```python
from build123d import *

# Parameters (mm, degrees)
BOSS_EXTRUDE1_DEPTH = 27.94
SKETCH2_R           = 3.175
BOSS_EXTRUDE2_DEPTH = 2.54
BOSS_EXTRUDE3_START = 3.81
SKETCH3_W           = 27.611756562
SKETCH3_H           = 25.107614127
SKETCH3_R           = 3.175
BOSS_EXTRUDE3_DEPTH = 3.81
SKETCH4_R           = 3.175
BOSS_EXTRUDE4_DEPTH = 18.954575182
SKETCH5_W           = 22.86
SKETCH5_H           = 21.59
CUT_EXTRUDE1_DEPTH  = 564.927995542


with BuildPart() as part:
    # Sketch1 → Boss-Extrude1 (new body)
    with BuildSketch(Plane.XY):
        with BuildLine():
            Line((-518.959059009, 348.633589309), (-527.727560082, 348.633589309))
            Line((-527.727560082, 348.633589309), (-527.727560082, 323.525975182))
            Line((-527.727560082, 323.525975182), (-500.11580352, 323.525975182))
            Line((-500.11580352, 323.525975182), (-500.11580352, 330.828951218))
            Line((-500.11580352, 330.828951218), (-503.31589155, 328.989459324))
            ThreePointArc((-503.31589155, 328.989459324), (-505.910190066, 327.86159111), (-508.689794246, 327.335975182))
            ThreePointArc((-508.689794246, 327.335975182), (-520.655570716, 333.67086151), (-520.107560082, 347.198990562))
            ThreePointArc((-520.107560082, 347.198990562), (-519.559291988, 347.937090778), (-518.959059009, 348.633589309))
        make_face()
    extrude(amount=-BOSS_EXTRUDE1_DEPTH)

    # Sketch2 → Boss-Extrude2 (add)
    with BuildSketch(Plane(origin=(0, 0, -25.4), x_dir=(-1, 0, 0), z_dir=(0, 0, -1))):
        with BuildLine():
            Line((500.11580352, 330.828951218), (500.11580352, 348.633589309))
            Line((500.11580352, 348.633589309), (518.959059009, 348.633589309))
            ThreePointArc((518.959059009, 348.633589309), (519.579835197, 332.088638139), (503.31589155, 328.989459324))
            Line((503.31589155, 328.989459324), (500.11580352, 330.828951218))
        make_face()
        with Locations(Location((509.64503004, 340, 0), (0, 0, 180))):
            Circle(SKETCH2_R, mode=Mode.SUBTRACT)
    extrude(amount=BOSS_EXTRUDE2_DEPTH)

    # Sketch3 → Boss-Extrude3 (add)
    with BuildSketch(Plane.XY.offset(BOSS_EXTRUDE3_START)):
        with Locations((-513.921681801, 336.079782246)):
            Rectangle(SKETCH3_W, SKETCH3_H)
        with Locations((-509.64503004, 340)):
            Circle(SKETCH3_R, mode=Mode.SUBTRACT)
    extrude(amount=-BOSS_EXTRUDE3_DEPTH)

    # Sketch4 → Boss-Extrude4 (add)
    with BuildSketch(Plane(origin=(0, 323.525975182, 0), x_dir=(1, 0, 0), z_dir=(0, 1, 0))):
        Polygon((-562.359793246, 33.660212868), (-511.559810801, 33.702445144), (-511.559793246, -29.839787132), (-562.359793246, -29.839787132), align=None)
        with Locations(Location((-539.26913234, -22.159639935, 0), (0, 0, 270))):
            Circle(SKETCH4_R, mode=Mode.SUBTRACT)
        with Locations(Location((-554.645069674, 26.257511479, 0), (0, 0, 270))):
            Circle(SKETCH4_R, mode=Mode.SUBTRACT)
    extrude(amount=-BOSS_EXTRUDE4_DEPTH)

    # Sketch5 → Cut-Extrude1 (cut, through all)
    with BuildSketch(Plane(origin=(0, 323.525975182, 0), x_dir=(1, 0, 0), z_dir=(0, 1, 0))):
        with Locations((-550.929793246, 0.005212868)):
            Rectangle(SKETCH5_W, SKETCH5_H)
    extrude(amount=-CUT_EXTRUDE1_DEPTH, mode=Mode.SUBTRACT)


solid = part.part
```
Geometry: final body of the model. Coordinates: model frame, mm. A direction names the side the tool comes from. Round coordinates to 2 decimals unless told otherwise and drop trailing zeros. Order: outer loops, then holes, each group sorted by start corner. A loop starts at its lowest first (then second) coordinate and runs counter-clockwise, first axis right, second up. Notation, with made-up numbers: M 32.25,77.25 L 83.25,77.25 A20 ccw 83.25,108.25 Z; hole C -37,70 d10. An arc over 180 degrees is marked long. One line per item, written item: value.
(1) Cut plane B-B (z = -2.5). Return the cut outline in (x, y).
Result sheet:
outline: M -539.5,304.57 L -511.56,304.57 L -511.56,323.53 L -500.12,323.53 L -500.12,330.83 L -503.32,328.99 A12.7 cw -518.96,348.63 L -527.73,348.63 L -527.73,323.53 L -539.5,323.53 Z
(2) Reachability of faces 1 (the flat face through (-539.5, 314, 0)), 2 (the flat face through (-514, 336, 3.81)), 3 (the flat face through (-527.728, 336, -12)), 4 (the flat face through (-501.693, 329.922, -12.522)) from +Z, -Z, +X, -X, +Y, -Y: full face, straight path, thin tool, end or side. Return the list, or none.
Result sheet:
face 1: -X, +Y, -Y
face 2: +Z, +X, -X, +Y
face 3: +Z, -Z, -X, +Y
face 4: +Y
(3) Line query: probe 1 along Z at (x, y) = (-542, 312.5); probe 2 along X at (y, z) = (317, -26); probe 3 along X at (y, z) = (340, 2.4). Output: solid intervals per line, ascending. Write a range as [from, to].
Result sheet:
probe 1: [-33.68, -10.8], [10.79, 20.54], [23.78, 29.84]
probe 2: [-562.36, -557.81], [-551.48, -511.56]
probe 3: [-527.73, -512.82], [-506.47, -500.12]
(4) Cut plane D-D (y = 319). Return the cut outline in (x, z) (3 decimals), and give its area (3 significant figures).
Result sheet:
outline: M -562.36,-33.66 L -511.56,-33.702 L -511.56,29.84 L -562.36,29.84 L -562.36,10.79 L -539.5,10.79 L -539.5,-10.8 L -562.36,-10.8 Z; hole C -554.645,-26.258 d6.35; hole C -539.269,22.16 d6.35
area: 2,670 mm2
(5) Pin query (flat end, axial travel): P1, Ø15, axis at y = 318.5, z = 1.5, coming from the -X side; P2, Ø1.5, axis at x = -548.5, z = -16, coming from the +Y side; P3, Ø23.5, axis at x = -509.5, y = 338.5, coming from the -Z side. Return the tip coordinate at first contact, or that it passes through.
Result sheet:
P1: x = -539.5
P2: y = 323.53
P3: z = -27.94
(6) Pull-direction query (X, two-part tool) for faces 5 (the cylindrical face through (-506.712, 341.216, -26.652)), 6 (the cylindrical face through (-542.1, 314.2, 23.6)), 7 (the flat face through (-551, 314, -10.8)), 8 (the flat face through (-511.56, 314, -2)); classes: pulls with the +X half, pulls with the -X half, needs draft (parallel to the pull), parting line crosses it, or undercut.
Result sheet:
face 5: undercut
face 6: undercut
face 7: needs draft
face 8: pulls with the +X half
(7) Cut plane A-A (y = 340). Return the cut outline in (x, z), and give its area (3 significant figures).
Result sheet:
outline: M -527.73,-27.94 L -512.82,-27.94 L -512.82,-25.4 L -522.35,-25.4 L -522.35,0 L -512.82,0 L -512.82,3.81 L -527.73,3.81 Z; M -506.47,-27.94 L -500.12,-27.94 L -500.12,-25.4 L -506.47,-25.4 Z; M -506.47,0 L -500.12,0 L -500.12,3.81 L -506.47,3.81 Z
area: 272 mm2
(8) Cut plane C-C (z = 23). Return the cut outline in (x, y), and give its area (3 significant figures).
Result sheet:
outline: M -562.36,304.57 L -542.33,304.57 L -542.33,323.53 L -562.36,323.53 Z; M -536.21,304.57 L -511.56,304.57 L -511.56,323.53 L -536.21,323.53 Z
area: 847 mm2
